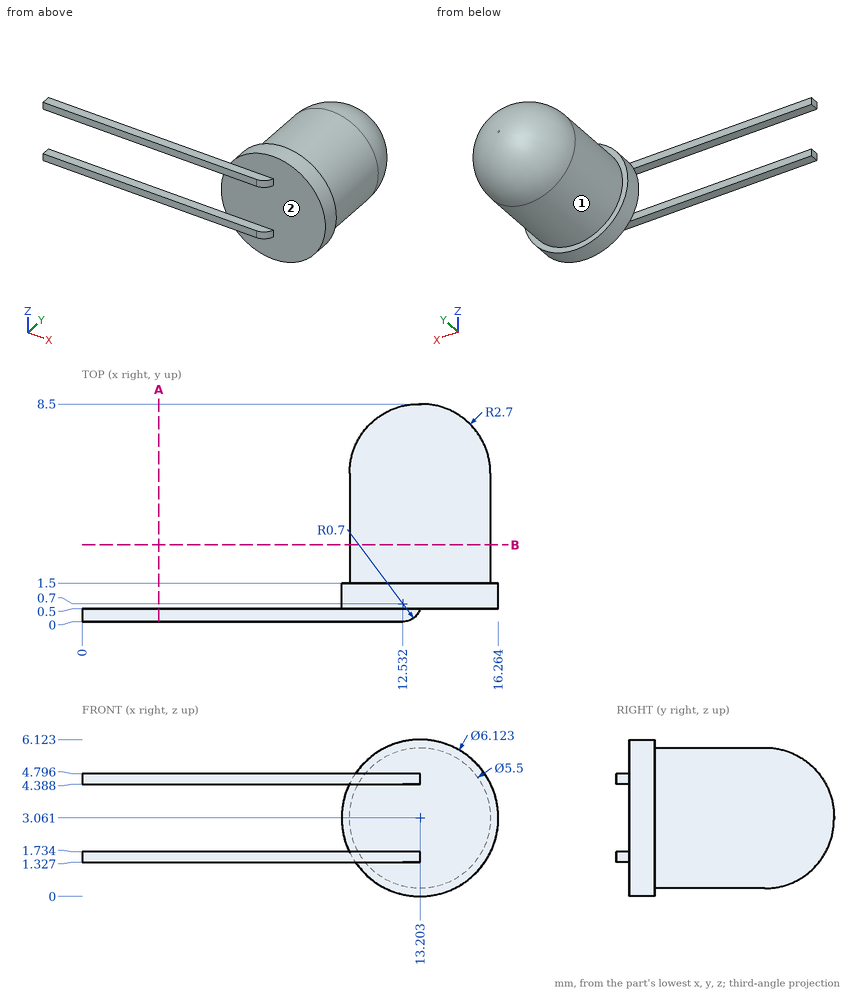
The drawing under review shows one solid part. Ordinate dimensions are in mm from its lowest x, y, z. Round coordinates to 2 decimals unless told otherwise and drop trailing zeros. Write each loop counter-clockwise with the first axis right and the second up, starting at its lowest first coordinate (ties: lowest second). Pieces come first, ordered by that corner, then holes. Notation, with made-up numbers: (-33.5, 8) - (-9.5, 8) arc R19 cw to (-9.5, 26) - close; hole circle Ø7 at (-11.5, -29.5). An arc over 180 degrees is marked (long way). One line per question, with ' | ' between items.
Item 1: For P1, Ø2, axis at y = 7, z = 2, coming from the +X side (1 decimal); P2, Ø1.5, axis at y = 6, z = 1.5, coming from the +X side; P3, Ø1, axis at y = 3.5, z = 4, coming from the -X side, all flat-tipped, find the tip position at first contact; note any pin that passes through.
Resolved:
P1: stops at x = 15.9 | P2: stops at x = 15.83 | P3: stops at x = 10.49
Item 2: The part is to be moulded in two halves that separate along Z. For the marked faces 1 and 2, say which applies: pulls with the +Z half, pulls with the -Z half, needs draft (parallel to the pull), parting line crosses it, or undercut.
Resolved:
face 1: parting line crosses it | face 2: undercut
Item 3: Add section B-B, the plane y = 3. Give the boundary of the cut face in (x, z).
Resolved:
outline: circle Ø5.5 at (13.2, 3.06)
Item 4: Add section A-A, the plane x = 3. Give the boundary of the cut face in (y, z) (1 decimal).
Resolved:
outline: (0, 1.3) - (0.5, 1.3) - (0.5, 1.7) - (0, 1.7) - close; (0, 4.4) - (0.5, 4.4) - (0.5, 4.8) - (0, 4.8) - close
Item 5: To check wall thickness, follow probe 1 along Z at (x, y) = (13.25, 2.5); probe 2 along Y at (x, z) = (1, 4.5); probe 3 along X at (y, z) = (1.75, 5.5) (1 decimal). State the ranges of each line that lie inside material, in increasing order.
Resolved:
probe 1: z = 0.31 to 5.81 | probe 2: y = 0 to 0.5 | probe 3: x = 11.9 to 14.5
